Autodesk Inventor part; units mm, degrees
ref_plane "Work Plane2" through (-27, 9, 0) normal (1, 0, 0) x (0, 1, 0)
ref_plane "XY Plane" through (0, 0, 0) normal (0, 0, 1) x (1, 0, 0)
sketch "Sketch3" plane through (0, 0, 0) normal (1, 0, 0) x (0, 1, 0)
  line L0 (63.5252, 0) -> (0, 0) construction
  line L1 (0, -8) -> (0, -27)
  line L2 (0, -27) -> (18, -27)
  line L3 (18, -27) -> (18, -12.4)
  line L4 (9, -8) -> (9, -12.4)
  line L5 (9, -12.4) -> (18, -12.4)
  line L6 (9, -8) -> (5, -8)
  line L7 (5, -8) -> (5, 0)
  line L8 (0, -8) -> (0, 0)
  line L9 (5, 0) -> (0, 0)
  dimension "d15" = 18
  dimension "d18" = 9
  dimension "d32" = 27
  dimension "d33" = 12.4
  dimension "d54" = 4
  dimension "d56" = 8
revolve "Revolution1" add sketch "Sketch3" angle 360 about axis through (0, 63.5252, 0) along (0, -1, 0)
fillet "Fillet2" radius 1 2 edges at (0, 18, 27) (0, 0, 27)
ref_plane "Work Plane2" through (-27, 9, 0) normal (1, 0, 0) x (0, 1, 0)
sketch "Sketch4" plane through (-27, 9, 0) normal (1, 0, 0) x (0, 1, 0)
  line L0 (-9, 0) -> (10.8256, 0) construction
  line L1 (-3.75, 3.75) -> (3.75, 3.75)
  line L2 (3.75, 3.75) -> (3.75, -3.75)
  line L3 (3.75, -3.75) -> (-3.75, -3.75)
  line L4 (-3.75, -3.75) -> (-3.75, 3.75)
  line L5 (-3.75, 3.75) -> (3.75, -3.75) construction
  line L6 (3.75, 3.75) -> (-3.75, -3.75) construction
  line L7 (9, 26) -> (9, -26)
  point P0 (0, 0)
  dimension "d21" = 7.5
  dimension "d22" = 7.5
  dimension "d55" = 9
extrude "Extrusion3" cut sketch "Sketch4" along normal blind 10
pattern_circular "Circular Pattern2" count 3 over 360 about axis through (0, 13.5, 0) along (0, -1, 0) of "Extrusion3"
sketch "Sketch9" plane through (0, 18, 0) normal (0, 1, 0) x (1, 0, 0)
  circle A0 centre (0, -22.4737) radius 3.5
  point P0 (0, 0)
  dimension "d57" = 7
extrude "Extrusion7" cut sketch "Sketch9" against normal blind 2.4
ref_plane "Work Plane4" through (0, 9, 0) normal (0, 1, 0) x (-1, 0, 0)
split "Split1" plane through (0, 9, 0) removes the side toward (0, -1, 0)
properties part number "BasePaletas"
The listing builds one solid part. Answer for the finished solid, in the listing's coordinates (mm). A direction names the side the tool comes from. Give positions to 0.01 mm unless a question says otherwise; leave off trailing zeros. Order: outer loops, then holes, each group sorted by start corner. A loop starts at its lowest first (then second) coordinate and runs counter-clockwise, first axis right, second up. Notation, with made-up numbers: M 55.25,80 L 100.25,80 A23 ccw 100.25,114 Z; hole C 60,69.25 d8. An arc over 180 degrees is marked long. Put each result on its own line as item: value. Start each with the question number.
Item 1: For a pull along X with two mould halves and no side action, classify faces 1 (the face through (-17, 11, 0)), 2 (the face through (23.954, 13.056, -12.459)), 3 (the face through (7.72, 10.85, -20.87)), 4 (the face through (-22, 11, 3.75)) as +X half, -X half, draft (parallel to the pull), parting line (faces both ways), or undercut.
Item 2: The part is cut by section B-B, the plane z = 0. Determine the outline of the cut face in (x, y).
Item 3: Which of the six approach directions +Z, -Z, +X, -X, +Y, -Y give full straight-line access (tool end or side, diameter ignored) to faces 5 (the face through (0, 15.6, 22)), 6 (the face through (8.545, 10.849, 14.696)), 7 (the face through (-22, 11, -3.75)), 8 (the face through (14.216, 10.901, -17.123)), 9 (the face through (14.216, 10.849, 17.123))?
Item 4: The part is cut by section C-C, the plane y = 13.5. Determine the outline of the cut face in (x, z), and give its area (3 significant figures).
Item 5: Flat-ended cylindrical pins translate along their axes: P1, Ø3, axis at x = -22.5, y = 11, coming from the -Z side; P2, Ø5, axis at y = 10.5, z = 7.5, coming from the -X side; P3, Ø2, axis at x = -13, y = 14, coming from the -Z side. Find the tip coordinate at first contact, or state that the pin passes through.
Item 6: Find the intervals of material crossed by line 1 along X through (y, z) = (15.75, 0); line 2 along X through (y, z) = (11.75, 0); line 3 along Z through (x, y) = (-8, 12.25), in increasing order.
Answer key:
1. face 1: -X half
1. face 2: parting line
1. face 3: undercut
1. face 4: draft
2. outline: M -27,12.75 L -17,12.75 L -17,9 L -12.4,9 L -12.4,18 L -26,18 A1 ccw -27,17 Z; M 12.4,9 L 27,9 L 27,17 A1 ccw 26,18 L 12.4,18 Z
3. face 5: +Y
3. face 6: -Y
3. face 7: -X, -Y
3. face 8: -Z, -Y
3. face 9: +Z, -Y
4. outline: C 0,0 d54; hole C 0,0 d24.8
4. area: 1,810 mm²
5. P1: stops at z = -16.97
5. P2: stops at x = -26.53
5. P3: stops at z = -24.19
6. line 1: x = -27 to -12.4, 12.4 to 27
6. line 2: x = -17 to -12.4, 12.4 to 27
6. line 3: z = -25.79 to -9.47, 9.47 to 25.79
